from build123d import *

# Parameters (mm, degrees)
SKETCH1_W             = 32
SKETCH1_H             = 48
BOSS_EXTRUDE1_DEPTH   = 3
BOSS_EXTRUDE2_DEPTH   = 4
CHAMFER1_SIZE         = 1
CHAMFER1_SIZE2        = 7.115369722
CHAMFER1_PART_2_SIZE  = 1
CHAMFER1_PART_2_SIZE2 = 7.115369722
CHAMFER2_SIZE         = 1
CHAMFER2_SIZE2        = 7.115369722
CHAMFER2_PART_2_SIZE  = 1
CHAMFER2_PART_2_SIZE2 = 7.115369722
SKETCH4_W             = 13.6
SKETCH4_H             = 2
CUT_EXTRUDE2_DEPTH    = 7
CHAMFER4_SIZE         = 2.5
CHAMFER4_SIZE2        = 2.979383981
CHAMFER4_PART_2_SIZE  = 2.5
CHAMFER4_PART_2_SIZE2 = 2.979383981
CHAMFER5_SIZE         = 2.5
SKETCH5_W             = 45.346149297
SKETCH5_H             = 21.744132288
CUT_EXTRUDE3_DEPTH    = 10


with BuildPart() as part:
    # Sketch1 → Boss-Extrude1 (new body)
    with BuildSketch(Plane(origin=(0, 0, 0), x_dir=(1, 0, 0), z_dir=(0, 1, 0))):
        Rectangle(SKETCH1_W, SKETCH1_H)
    extrude(amount=BOSS_EXTRUDE1_DEPTH)

    # Sketch2 → Boss-Extrude2 (add)
    with BuildSketch(Plane.XZ):
        Polygon((-13.95, -21.95), (-11.95, -21.95), (-11.95, -19.95), (-11.95, 19.95), (-6.8, 19.95), (-6.8, 21.95), (-13.95, 21.95), align=None)
        Polygon((11.95, -19.95), (11.95, -21.95), (13.95, -21.95), (13.95, 21.95), (6.8, 21.95), (6.8, 19.95), (11.95, 19.95), align=None)
    extrude(amount=BOSS_EXTRUDE2_DEPTH)

    # Chamfer1
    chamfer1_edges = [part.edges().sort_by_distance(p)[0] for p in [
        (0, 3, 24),
    ]]
    chamfer1_side = [part.faces().sort_by_distance(p)[0] for p in [
        (0, 1.5, 24),
    ]]
    chamfer(chamfer1_edges, length=CHAMFER1_SIZE, length2=CHAMFER1_SIZE2, reference=chamfer1_side[0])

    # Chamfer1 part 2
    chamfer1_part_2_edges = [part.edges().sort_by_distance(p)[0] for p in [
        (0, 3, -24),
    ]]
    chamfer1_part_2_side = [part.faces().sort_by_distance(p)[0] for p in [
        (0, 1.5, -24),
    ]]
    chamfer(chamfer1_part_2_edges, length=CHAMFER1_PART_2_SIZE, length2=CHAMFER1_PART_2_SIZE2, reference=chamfer1_part_2_side[0])

    # Chamfer2
    chamfer2_edges = [part.edges().sort_by_distance(p)[0] for p in [
        (16, 3, 0),
    ]]
    chamfer2_side = [part.faces().sort_by_distance(p)[0] for p in [
        (16, 1.439355758, 0),
    ]]
    chamfer(chamfer2_edges, length=CHAMFER2_SIZE, length2=CHAMFER2_SIZE2, reference=chamfer2_side[0])

    # Chamfer2 part 2
    chamfer2_part_2_edges = [part.edges().sort_by_distance(p)[0] for p in [
        (-16, 3, 0),
    ]]
    chamfer2_part_2_side = [part.faces().sort_by_distance(p)[0] for p in [
        (-16, 1.439355758, 0),
    ]]
    chamfer(chamfer2_part_2_edges, length=CHAMFER2_PART_2_SIZE, length2=CHAMFER2_PART_2_SIZE2, reference=chamfer2_part_2_side[0])

    # Sketch4 → Cut-Extrude2 (cut)
    with BuildSketch(Plane.XY.offset(24)):
        with Locations((0, 1)):
            Rectangle(SKETCH4_W, SKETCH4_H)
    extrude(amount=-CUT_EXTRUDE2_DEPTH, mode=Mode.SUBTRACT)

    # Chamfer4
    chamfer4_edges = [part.edges().sort_by_distance(p)[0] for p in [
        (16, 1, 24),
    ]]
    chamfer4_side = [part.faces().sort_by_distance(p)[0] for p in [
        (11.4, 1, 24),
    ]]
    chamfer(chamfer4_edges, length=CHAMFER4_SIZE, length2=CHAMFER4_SIZE2, reference=chamfer4_side[0])

    # Chamfer4 part 2
    chamfer4_part_2_edges = [part.edges().sort_by_distance(p)[0] for p in [
        (-16, 1, 24),
    ]]
    chamfer4_part_2_side = [part.faces().sort_by_distance(p)[0] for p in [
        (-16, 1, 0),
    ]]
    chamfer(chamfer4_part_2_edges, length=CHAMFER4_PART_2_SIZE, length2=CHAMFER4_PART_2_SIZE2, reference=chamfer4_part_2_side[0])

    # Chamfer5
    chamfer5_edges = [part.edges().sort_by_distance(p)[0] for p in [
        (16, 1, -24),
        (-16, 1, -24),
    ]]
    chamfer(chamfer5_edges, length=CHAMFER5_SIZE)

    # Sketch5 → Cut-Extrude3 (cut)
    with BuildSketch(Plane(origin=(0, 3, 0), x_dir=(1, 0, 0), z_dir=(0, 1, 0))):
        with Locations((0.997752906, 15.619993764)):
            Rectangle(SKETCH5_W, SKETCH5_H)
    extrude(amount=-CUT_EXTRUDE3_DEPTH, mode=Mode.SUBTRACT)


solid = part.part
Read the model definition and answer for the solid it produces. Units are mm, in the model's axes. A direction names the side the tool comes from. Round coordinates to 2 decimals unless told otherwise and drop trailing zeros. Write each loop counter-clockwise with the first axis right and the second up, starting at its lowest first coordinate (ties: lowest second). Pieces come first, ordered by that corner, then holes.
Q1. Find section A-A on y = -1.5. Determine the outline of the cut face in (x, z).
Values:
outline: (-13.95, -4.75) - (-11.95, -4.75) - (-11.95, 19.95) - (-6.8, 19.95) - (-6.8, 21.95) - (-13.95, 21.95) - close; (6.8, 19.95) - (11.95, 19.95) - (11.95, -4.75) - (13.95, -4.75) - (13.95, 21.95) - (6.8, 21.95) - close
Q2. Straight lines are drawn through the part: line 1 (X direction, y = -0.75, z = 12); line 2 (Y direction, x = -4, z = -2.5); line 3 (Z direction, x = -4, y = 0.5). For each, find the intervals that lie inside material, in ascending order.
Values:
line 1: x = -13.95 to -11.95, 11.95 to 13.95
line 2: y = 0 to 3
line 3: z = -4.75 to 17
Q3. Find section B-B on x = 7.5. Determine the outline of the cut face in (y, z), and give its area (3 significant figures).
Values:
outline: (-4, 19.95) - (0, 19.95) - (0, -4.75) - (3, -4.75) - (3, 16.88) - (2, 24) - (0, 24) - (0, 21.95) - (-4, 21.95) - close
area: 90.7 mm2
Q4. The mould has two halves that part along X. Classify faces 1 (the face through (-0.205, 2.507, 20.393)), 2 (the face through (0, 2, 21)), 3 (the face through (0, 0, 7)), 4 (the face through (13.95, -2, 8)): released by +X, released by -X, zero draft, split by the parting line, or undercut.
Values:
face 1: zero draft
face 2: undercut
face 3: undercut
face 4: released by +X
Q5. Find section D-D on y = 1.5. Determine the outline of the cut face in (x, z), and give its area (3 significant figures).
Values:
outline: (-16, -4.75) - (16, -4.75) - (16, 21.02) - (13.5, 24) - (6.8, 24) - (6.8, 17) - (-6.8, 17) - (-6.8, 24) - (-13.02, 24) - (-16, 21.5) - close
area: 817 mm2
Q6. Find section C-C on z = 13.5. Determine the outline of the cut face in (x, y).
Values:
outline: (-16, 0) - (-13.95, 0) - (-13.95, -4) - (-11.95, -4) - (-11.95, 0) - (11.95, 0) - (11.95, -4) - (13.95, -4) - (13.95, 0) - (16, 0) - (16, 2) - (8.88, 3) - (-8.88, 3) - (-16, 2) - close
Q7. Flat-ended cylindrical pins translate along their axes: P1, Ø1.2, axis at y = -2, z = 11, coming from the -X side; P2, Ø1.2, axis at y = -2.5, z = 8, coming from the +X side; P3, Ø2, axis at x = 9.5, y = -2, coming from the -Z side. Find the tip coordinate at first contact, or state that the pin passes through.
Values:
P1: stops at x = -13.95
P2: stops at x = 13.95
P3: stops at z = 19.95
Q8. A tool of negligible diameter and unlimited length cuts with its end or side. For faces 5 (the face through (-11.95, -2, 7)), 6 (the face through (10, -2, 21.95)), 7 (the face through (-13.95, -2, 9)), 8 (the face through (6.8, 0, 21)), from which of +Z, -Z, +X, -X, +Y, -Y can it reach the whole face along a straight path? Write none if from no direction.
Values:
face 5: -Z, -Y
face 6: +Z, +X, -X, -Y
face 7: +Z, -Z, -X, -Y
face 8: +Z, -Y
